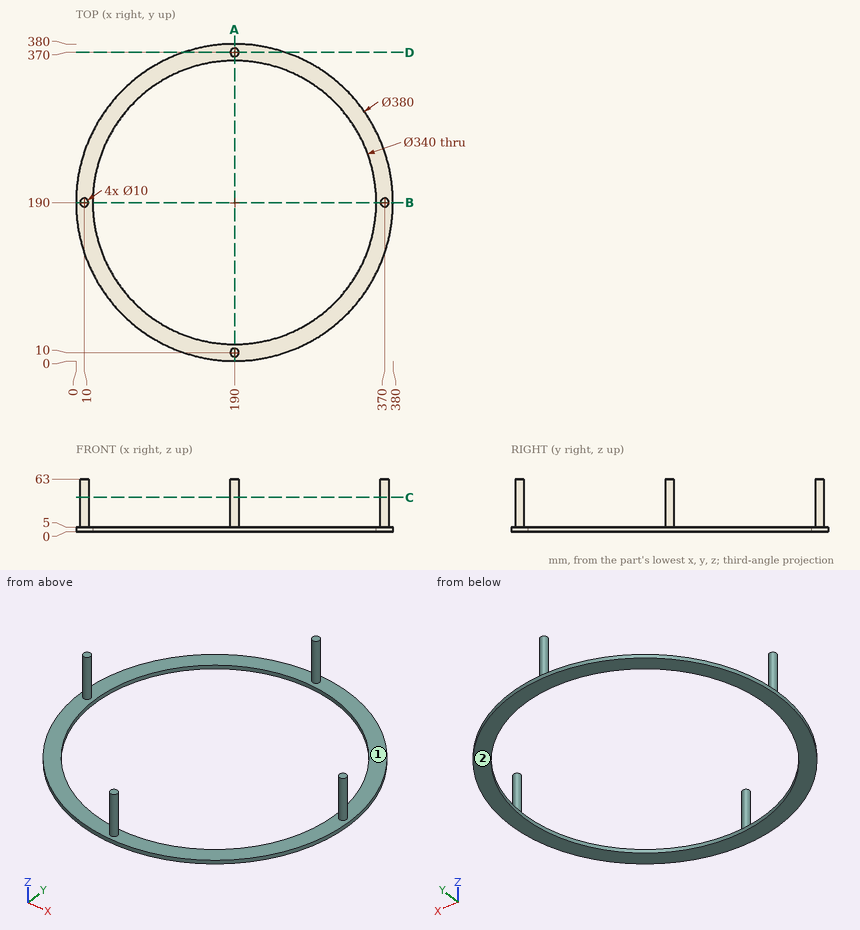
Part print with two shaded views. Sizes in mm from the minimum x, y, z corner. Round coordinates to 2 decimals unless told otherwise and drop trailing zeros. Write each loop counter-clockwise with the first axis right and the second up, starting at its lowest first coordinate (ties: lowest second). Pieces come first, ordered by that corner, then holes. Notation, with made-up numbers: (75, 42) -> (86, 42) arc R11 ccw to (86, 47) -> close; hole circle Ø7 at (43.25, 26). An arc over 180 degrees is marked (long way). Put each result on its own line as item: value.
Item 1: Slice it at A-A, the plane x = 190. Give the cut face in (y, z).
Here are the results:
outline: (0, 0) -> (20, 0) -> (20, 5) -> (15, 5) -> (15, 63) -> (5, 63) -> (5, 5) -> (0, 5) -> close; (360, 0) -> (380, 0) -> (380, 5) -> (375, 5) -> (375, 63) -> (365, 63) -> (365, 5) -> (360, 5) -> close
Item 2: Flat gauge pins, fed straight in: P1, Ø10, axis at x = 315, z = 9.5, coming from the -Y side; P2, Ø5, axis at x = 289.5, y = 324.5, coming from the -Z side. Where does each tip first touch, or does it go through?
Here are the results:
P1: stops at y = 45.03
P2: passes through
Item 3: Slice it at C-C, the plane z = 41. Give the cut face in (x, y), plus the area to 3 significant figures.
Here are the results:
outline: circle Ø10 at (10, 190); circle Ø10 at (190, 10); circle Ø10 at (190, 370); circle Ø10 at (370, 190)
area: 314 mm^2
Item 4: Wall check: probe 1 along Y at (x, z) = (190, 1.6); probe 2 along X at (y, z) = (186.5, 14.5). Give the ranges that are in metal, low to high. Write a range as from..to.
Here are the results:
probe 1: y = 0..20, 360..380
probe 2: x = 6.43..13.57, 366.43..373.57
Item 5: Two-plate mould, pull along Z, no slides. Class the marked faces 1 and 2: pulls with the +Z half, pulls with the -Z half, needs draft (parallel to the pull), parting line crosses it, or undercut.
Here are the results:
face 1: pulls with the +Z half
face 2: pulls with the -Z half
Item 6: Slice it at D-D, the plane y = 370. Give the cut face in (x, z).
Here are the results:
outline: (129.17, 0) -> (250.83, 0) -> (250.83, 5) -> (195, 5) -> (195, 63) -> (185, 63) -> (185, 5) -> (129.17, 5) -> close
